For this review, take the finished solid that the model builds, in its own axes (mm). Face numbers are marked on the shaded views. A direction names the side the tool comes from. Coordinates: 2 decimals unless noted, no trailing zeros. Loops run counter-clockwise (first coordinate to the right, second up) from the corner with the lowest first, then second, coordinate; pieces in that order, holes last. Notation, with made-up numbers: (40.5, 59) -> (45.5, 59) arc R8 cw to (45.5, 74) -> close; hole circle Ø4 at (46.5, 3). An arc over 180 degrees is marked (long way). One line per item, written item: value.
from build123d import *

# Parameters (mm, degrees)
F0_R     = 9.525
F1_DEPTH = 25.4
F3_DEPTH = 25.401
F4_DEPTH = 11.1252
F6_DEPTH = 12.7


with BuildPart() as f1:
    # F0 (on Front) → F1 (new body)
    with BuildSketch(Plane.XZ):
        Circle(F0_R)
    extrude(amount=F1_DEPTH)

    # F2 (on Front) → F3 (cut, through all)
    with BuildSketch(Plane.XZ):
        with BuildLine():
            ThreePointArc((-4.7625, 0), (-3.367596, -3.367596), (0, -4.7625))
            ThreePointArc((0, -4.7625), (3.367596, -3.367596), (4.7625, 0))
            ThreePointArc((4.7625, 0), (3.367596, 3.367596), (0, 4.7625))
            ThreePointArc((0, 4.7625), (-3.367596, 3.367596), (-4.7625, 0))
        make_face()
    extrude(amount=F3_DEPTH, mode=Mode.SUBTRACT)

    # F2 (on Front) → F4 (cut)
    with BuildSketch(Plane.XZ):
        with BuildLine():
            ThreePointArc((0, 4.7625), (3.367596, 3.367596), (4.7625, 0))
            Line((4.7625, 0), (4.7625, 4.7625))
            Line((4.7625, 4.7625), (0, 4.7625))
        make_face()
        with BuildLine():
            Line((-4.7625, 4.7625), (-4.7625, 0))
            ThreePointArc((-4.7625, 0), (-3.367596, 3.367596), (0, 4.7625))
            Line((0, 4.7625), (-4.7625, 4.7625))
        make_face()
        with BuildLine():
            Line((-4.7625, -4.7625), (0, -4.7625))
            ThreePointArc((0, -4.7625), (-3.367596, -3.367596), (-4.7625, 0))
            Line((-4.7625, 0), (-4.7625, -4.7625))
        make_face()
        with BuildLine():
            Line((0, -4.7625), (4.7625, -4.7625))
            Line((4.7625, -4.7625), (4.7625, 0))
            ThreePointArc((4.7625, 0), (3.367596, -3.367596), (0, -4.7625))
        make_face()
    extrude(amount=F4_DEPTH, mode=Mode.SUBTRACT)

    # F5 (on face) → F6 (cut)
    with BuildSketch(Plane.XZ.offset(25.4)):
        Polygon((3.666174, -6.35), (7.332348, 0), (3.666174, 6.35), (-3.666174, 6.35), (-7.332348, 0), (-3.666174, -6.35), align=None)
    extrude(amount=-F6_DEPTH, mode=Mode.SUBTRACT)


solid = f1.part
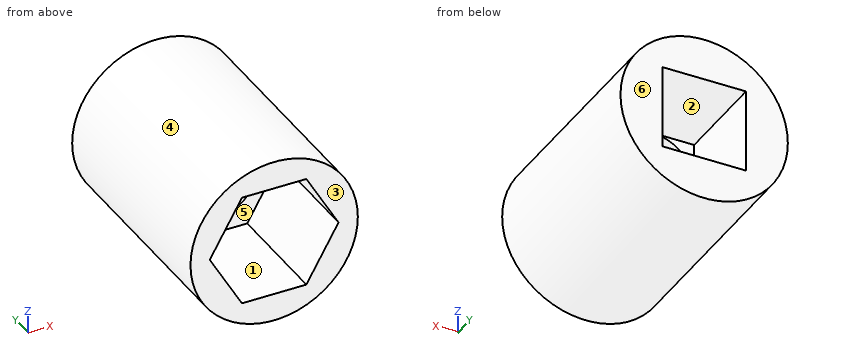
1. Insertion check: pin 1 Ø2.5 at (x, z) = (3, 2.5) entering from +Y; pin 2 Ø3 at (x, y) = (5, -20) entering from +Z; pin 3 Ø1 at (y, z) = (-10, 6.5) entering from +X. Each pin has a flat end and moves straight along its axis. Give the tip position at first contact, or say it passes through.
Return value:
pin 1: stops at y = -11.13
pin 2: stops at z = 8.86
pin 3: stops at x = 7.4
2. Take a section at A-A, the plane z = -4.25. Give the boundary of the cut face in (x, y).
Return value:
outline: (-8.52, -25.4) -> (-4.88, -25.4) -> (-4.88, -12.7) -> (-2.15, -12.7) -> (-2.15, -11.13) -> (-4.76, -11.13) -> (-4.76, 0) -> (-8.52, 0) -> close; (2.15, -12.7) -> (4.88, -12.7) -> (4.88, -25.4) -> (8.52, -25.4) -> (8.52, 0) -> (4.76, 0) -> (4.76, -11.13) -> (2.15, -11.13) -> close
3. For the marked faces 1, 2 and 3, list the 3-axis set-ups (+Z, -Z, +X, -X, +Y, -Y) from which the entire face can be reached by the end or side of a thin tool; tool diameter is ignored.
Return value:
face 1: -Y
face 2: +Y
face 3: +Z, -Z, +X, -X, -Y
4. To check wall thickness, follow probe 1 along X at (y, z) = (-5.25, 3.5); probe 2 along Z at (x, y) = (3.25, -12); probe 3 along X at (y, z) = (-17, 2). State the ranges of each line that lie inside material, in increasing order. Write a range as from..to.
Return value:
probe 1: x = -8.86..-4.76, 4.76..8.86
probe 2: z = -8.95..-3.48, 3.48..8.95
probe 3: x = -9.31..-6.18, 6.18..9.31
5. Take a section at B-B, the plane y = -14.5. Give the boundary of the cut face in (x, z) (3 decimals), and give its area (3 significant figures).
Return value:
outline: circle Ø19.05 at (0, 0); hole (-7.332, 0) -> (-3.666, -6.35) -> (3.666, -6.35) -> (7.332, 0) -> (3.666, 6.35) -> (-3.666, 6.35) -> close
area: 145 mm2
6. Take a section at C-C, the plane x = 6. Give the boundary of the cut face in (y, z), and give its area (3 significant figures).
Return value:
outline: (-25.4, -7.4) -> (0, -7.4) -> (0, 7.4) -> (-25.4, 7.4) -> (-25.4, 2.31) -> (-12.7, 2.31) -> (-12.7, -2.31) -> (-25.4, -2.31) -> close
area: 317 mm2
7. The part is to be moulded in two halves that separate along X. For the marked faces 4, 5 and 6, say which applies: pulls with the +X half, pulls with the -X half, needs draft (parallel to the pull), parting line crosses it, or undercut.
Return value:
face 4: parting line crosses it
face 5: undercut
face 6: needs draft
